```python
from build123d import *

# Parameters (mm, degrees)
F0_R     = 3.125
F1_DEPTH = 3.175
F2_W     = 15
F2_H     = 3.175
F2_W_2   = 7.5
F3_DEPTH = 25


# Not quite as in the source:
# - a feature names something its author has since deleted; it is built from what else it names


with BuildPart() as f1:
    # F0 (on Top) → F1 (new body)
    with BuildSketch(Plane.XY):
        with BuildLine():
            ThreePointArc((40, -50.3277523465), (57.898111611, -27.9408541051), (64.2875, 0))
            ThreePointArc((64.2875, 0), (57.898111611, 27.9408541051), (40, 50.3277523465))
            Line((40, 50.3277523465), (40, -50.3277523465))
        make_face()
        with BuildLine():
            Line((40, -50.3277523465), (40, 50.3277523465))
            ThreePointArc((40, 50.3277523465), (5.1835564074, 64.0781819282), (-31.390378499, 56.1028234043))
            ThreePointArc((-31.390378499, 56.1028234043), (-37.8178330459, 38.5576092221), (-40, 20))
            Line((-40, 20), (-40, -20))
            ThreePointArc((-40, -20), (-37.8178330459, -38.5576092221), (-31.390378499, -56.1028234043))
            ThreePointArc((-31.390378499, -56.1028234043), (5.1835564074, -64.0781819282), (40, -50.3277523465))
        make_face()
        Circle(F0_R, mode=Mode.SUBTRACT)
        with BuildLine():
            ThreePointArc((-31.390378499, 56.1028234043), (5.1835564074, 64.0781819282), (40, 50.3277523465))
            Line((40, 50.3277523465), (40, 100))
            ThreePointArc((40, 100), (-1.9033061205, 88.1477287675), (-31.390378499, 56.1028234043))
        make_face()
        with BuildLine():
            Line((40, -100), (40, -50.3277523465))
            ThreePointArc((40, -50.3277523465), (5.1835564074, -64.0781819282), (-31.390378499, -56.1028234043))
            ThreePointArc((-31.390378499, -56.1028234043), (-1.9033061205, -88.1477287675), (40, -100))
        make_face()
        with BuildLine():
            ThreePointArc((-40, 20), (-37.8178330459, 38.5576092221), (-31.390378499, 56.1028234043))
            ThreePointArc((-31.390378499, 56.1028234043), (-64.2875, 0), (-31.390378499, -56.1028234043))
            ThreePointArc((-31.390378499, -56.1028234043), (-37.8178330459, -38.5576092221), (-40, -20))
            Line((-40, -20), (-40, 20))
        make_face()
    extrude(amount=F1_DEPTH)

    # F2 (on face) → F3 (cut)
    with BuildSketch(Plane.XY.offset(3.175)):
        with Locations((-4, 38.4125)):
            Rectangle(F2_W, F2_H)
        with Locations((13.25, 38.4125)):
            Rectangle(F2_W_2, F2_H)
        with Locations((20.75, 38.4125)):
            Rectangle(F2_W_2, F2_H)
        with Locations((38, 38.4125)):
            Rectangle(F2_W, F2_H)
        with Locations((-4, -38.4125)):
            Rectangle(F2_W, F2_H)
        with Locations((20.75, -38.4125)):
            Rectangle(F2_W_2, F2_H)
        with Locations((38, -38.4125)):
            Rectangle(F2_W, F2_H)
        with Locations((13.25, -38.4125)):
            Rectangle(F2_W_2, F2_H)
        with Locations((-25, -38.4125)):
            Rectangle(F2_W, F2_H)
        with Locations((-25, 38.4125)):
            Rectangle(F2_W, F2_H)
    extrude(amount=-F3_DEPTH, mode=Mode.SUBTRACT)


solid = f1.part
```
Source: CAD feature listing. Evaluate the final solid. Frame: model axes, mm. Round coordinates to 2 decimals unless told otherwise and drop trailing zeros. Loops run counter-clockwise (first coordinate to the right, second up) from the corner with the lowest first, then second, coordinate; pieces in that order, holes last. Notation, with made-up numbers: M 1,33.25 L 18,33.25 A18 ccw 18,40.25 Z; hole C 40,11 d10. An arc over 180 degrees is marked long. Use a Markdown table: item, result. Add a question column.
1. Section query B-B on x = 0. Return the cut outline in (y, z) (3 decimals).
2. Contact query for flat-ended pins moving along their axis: P1, Ø1.6, axis at y = 38, z = 2, coming from the +X side; P2, Ø1.6, axis at x = 34.5, z = 2, coming from the -Y side; P3, Ø1.6, axis at y = -67.5, z = 2.5, coming from the +X side; P4, Ø10, axis at x = 46, y = 57.5, coming from the -Z side. Output: stop coordinate, or through.
3. Section query C-C on y = 44. Return the cut outline in (x, z) (3 decimals), then the cut area to 3 significant figures.
4. Section query D-D on x = -52. Return the cut outline in (y, z) (3 decimals).
5. Section query A-A on z = 1.8. Give the number of separate pieces and of enclosed holes in the cut face, then the cut area to 3 significant figures.
6. Line query: line 1 (Y direction, x = 0, z = 2.35) (3 decimals); line 2 (Y direction, x = 10.5, z = 1.05) (3 decimals); line 3 (Y direction, x = 20.5, z = 2.1) (3 decimals). Output: solid intervals per line, ascending.
Reported:
| question | item | result |
|---|---|---|
| 1 | outline | M -89.282,0 L -40,0 L -40,3.175 L -89.282,3.175 Z; M -36.825,0 L -3.125,0 L -3.125,3.175 L -36.825,3.175 Z; M 3.125,0 L 36.825,0 L 36.825,3.175 L 3.125,3.175 Z; M 40,0 L 89.282,0 L 89.282,3.175 L 40,3.175 Z |
| 2 | P1 | stops at x = 52.43 |
| 2 | P2 | stops at y = -99.86 |
| 2 | P3 | stops at x = 40 |
| 2 | P4 | passes through |
| 3 | outline | M -46.871,0 L 46.871,0 L 46.871,3.175 L -46.871,3.175 Z |
| 3 | area | 298 mm² |
| 4 | outline | M -37.801,0 L 37.801,0 L 37.801,3.175 L -37.801,3.175 Z |
| 5 | separate pieces | 1 |
| 5 | enclosed holes | 9 |
| 5 | area | 16,400 mm² |
| 6 | line 1 | y = -89.282 to -40, -36.825 to -3.125, 3.125 to 36.825, 40 to 89.282 |
| 6 | line 2 | y = -94.362 to -40, -36.825 to 36.825, 40 to 94.362 |
| 6 | line 3 | y = -97.587 to -40, -36.825 to 36.825, 40 to 97.587 |
